Model file for the job. Use its own axes, mm. A direction names the side the tool comes from. Round coordinates to 2 decimals unless told otherwise and drop trailing zeros. Write each loop counter-clockwise with the first axis right and the second up, starting at its lowest first coordinate (ties: lowest second). Pieces come first, ordered by that corner, then holes. Notation, with made-up numbers: (-5, 31.5) - (2, 31.5) arc R24 ccw to (2, 70.5) - close; hole circle Ø3 at (80.5, 66.25). An arc over 180 degrees is marked (long way). Answer as a JSON object with one key per item and string values. Group by question number.
from build123d import *

# Parameters (mm, degrees)
F1_DEPTH = 40
F3_DEPTH = 2
F4_R     = 15


with BuildPart() as f1:
    # F0 (on Top) → F1 (new body)
    with BuildSketch(Plane.XY):
        Polygon((-20, -3.65), (-12, -3.65), (-12, -1.65), (-18, -1.65), (-18, 1.65), (20, 1.65), (20, 3.65), (-20, 3.65), align=None)
    extrude(amount=F1_DEPTH)

    # F2 (on face) → F3 (cut, through all)
    with BuildSketch(Plane(origin=(0, 3.65, 0), x_dir=(-1, 0, 0), z_dir=(0, 1, 0))):
        with BuildLine():
            Line((-12.75, 16.75), (-10.799671, 16.75))
            Line((-10.799671, 16.75), (-7, 16.75))
            Line((-7, 16.75), (-7, 23.25))
            Line((-7, 23.25), (-10.799671, 23.25))
            Line((-10.799671, 23.25), (-12.75, 23.25))
            ThreePointArc((-12.75, 23.25), (-16, 20), (-12.75, 16.75))
        make_face()
        with BuildLine():
            Line((-7, 16.75), (-10.799671, 16.75))
            ThreePointArc((-10.799671, 16.75), (-2, 20), (-10.799671, 23.25))
            Line((-10.799671, 23.25), (-7, 23.25))
            Line((-7, 23.25), (-7, 16.75))
        make_face()
    extrude(amount=-F3_DEPTH, mode=Mode.SUBTRACT)

    # F4
    f4_edges = [f1.edges().sort_by_distance(p)[0] for p in [
        (20, 2.65, 40),
        (20, 2.65, 0),
    ]]
    fillet(f4_edges, radius=F4_R)


solid = f1.part
(1) Drill centre lines: line 1 (Y direction, x = -14.5, z = 26.5); line 2 (X direction, y = 2.2, z = 20); line 3 (Y direction, x = -5.5, z = 36). Where is each one in solid material? Low to high. Write a range as from..to.
(2) Slice it at D-D (x = 9). Write the cut outline in (y, z).
(3) Slice it at B-B (x = -15). Write the cut outline in (y, z).
(4) 3-axis set-ups, long thin cutter, end or side, ignore diameter. For faces 1 (the flat face through (12, 3, 23.25)), 2 (the flat face through (-15, -1.65, 20)), 3 (the flat face through (-12, -3, 20)): which of +Z, -Z, +X, -X, +Y, -Y reach the whole face in a straight line?
(5) Slice it at A-A (z = 20). Write the cut outline in (x, y).
(6) Flat gauge pins, fed straight in: pin 1 (1.6 mm diameter, centred on x = 12, y = 3, fed in from +Z); pin 2 (16 mm diameter, centred on x = 7, z = 20, fed in from -Y); pin 3 (0.6 mm diameter, centred on y = -3, z = 18, fed in from +X). Where does each tip first touch, or does it go through?
(7) Slice it at C-C (z = 16). Write the cut outline in (x, y).
(8) Pull direction Y, two halves, no side cores. Call faces 4 (the flat face through (-18, 0, 20)), 5 (the flat face through (0, 3.65, 20)), 6 (the cylindrical face through (16, 3, 20)): pulls with the +Y half, pulls with the -Y half, needs draft (parallel to the pull), parting line crosses it, or undercut.
Answer:
{
 "1": {"line 1": "-3.65..-1.65, 1.65..3.65", "line 2": "-20..2, 16..20", "line 3": "1.65..3.65"},
 "2": {"outline": "(1.65, 0.54) - (3.65, 0.54) - (3.65, 15.42) - (1.65, 15.42) - close; (1.65, 24.58) - (3.65, 24.58) - (3.65, 39.46) - (1.65, 39.46) - close"},
 "3": {"outline": "(-3.65, 0) - (-1.65, 0) - (-1.65, 40) - (-3.65, 40) - close; (1.65, 0) - (3.65, 0) - (3.65, 40) - (1.65, 40) - close"},
 "4": {"face 1": "+Y, -Y", "face 2": "+Z, -Z, +X", "face 3": "+Z, -Z, +X, -Y"},
 "5": {"outline": "(-20, -3.65) - (-12, -3.65) - (-12, -1.65) - (-18, -1.65) - (-18, 1.65) - (2, 1.65) - (2, 3.65) - (-20, 3.65) - close; (16, 1.65) - (20, 1.65) - (20, 3.65) - (16, 3.65) - close"},
 "6": {"pin 1": "z = 38.66", "pin 2": "y = 1.65", "pin 3": "x = -12"},
 "7": {"outline": "(-20, -3.65) - (-12, -3.65) - (-12, -1.65) - (-18, -1.65) - (-18, 1.65) - (4, 1.65) - (4, 3.65) - (-20, 3.65) - close; (10, 1.65) - (20, 1.65) - (20, 3.65) - (10, 3.65) - close"},
 "8": {"face 4": "undercut", "face 5": "pulls with the +Y half", "face 6": "needs draft"}
}
